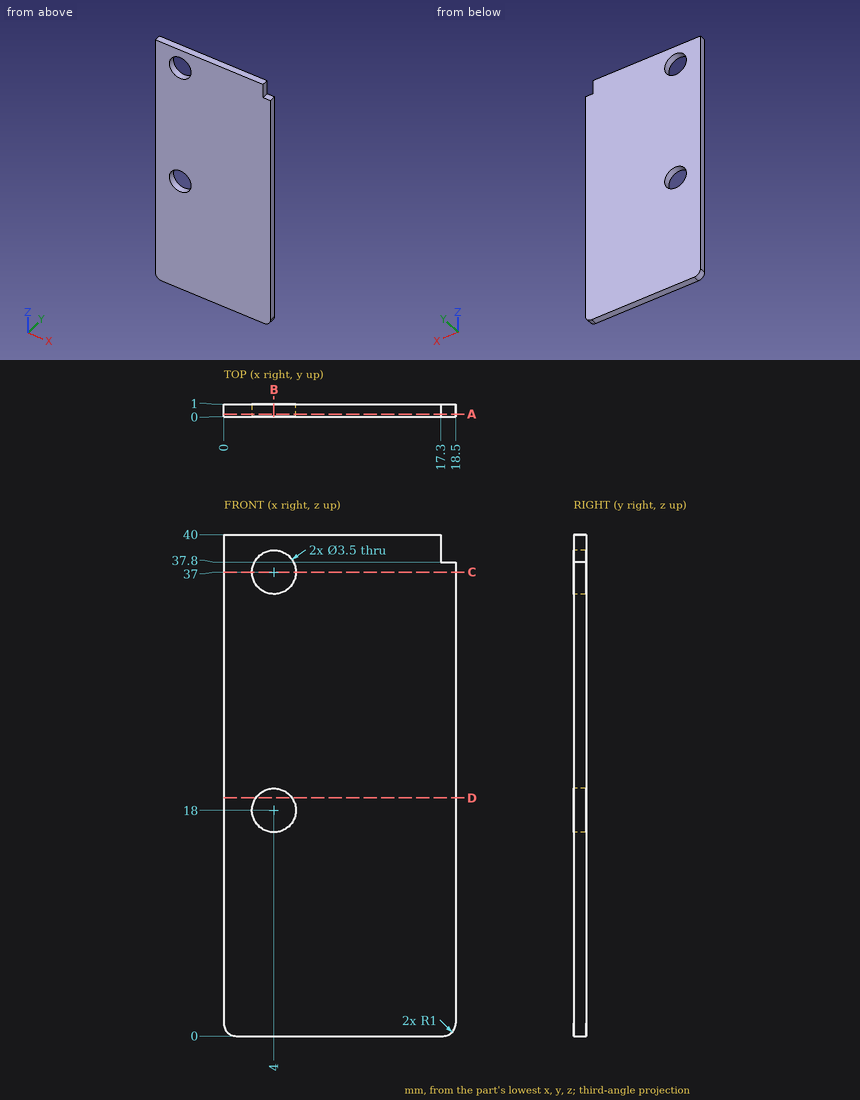
Print and shaded views of the part. All mm, measured from the part's lowest x, y and z. Give positions to 0.01 mm unless a question says otherwise; leave off trailing zeros. Write each loop counter-clockwise with the first axis right and the second up, starting at its lowest first coordinate (ties: lowest second). Pieces come first, ordered by that corner, then holes. Notation, with made-up numbers: (-13, 24) -> (30, 24) arc R11 ccw to (30, 34) -> close; hole circle Ø3 at (0.25, -2.5). An arc over 180 degrees is marked (long way). Write item = value, one per line.
(1) Slice it at B-B, the plane x = 4. Give the cut face in (y, z), then the cut area to 3 significant figures.
Determined:
outline = (0, 0) -> (1, 0) -> (1, 16.25) -> (0, 16.25) -> close; (0, 19.75) -> (1, 19.75) -> (1, 35.25) -> (0, 35.25) -> close; (0, 38.75) -> (1, 38.75) -> (1, 40) -> (0, 40) -> close
area = 33.0 mm2
(2) Slice it at D-D, the plane z = 19. Give the cut face in (x, y).
Determined:
outline = (0, 0) -> (2.56, 0) -> (2.56, 1) -> (0, 1) -> close; (5.44, 0) -> (18.5, 0) -> (18.5, 1) -> (5.44, 1) -> close
(3) Slice it at A-A, the plane y = 0.2. Give the cut face in (x, z), then the cut area to 3 significant figures.
Determined:
outline = (0, 1) arc R1 ccw to (1, 0) -> (17.5, 0) arc R1 ccw to (18.5, 1) -> (18.5, 37.8) -> (17.3, 37.8) -> (17.3, 40) -> (0, 40) -> close; hole circle Ø3.5 at (4, 18); hole circle Ø3.5 at (4, 37)
area = 718 mm2
(4) Flat gauge pin, fed straight in: P1, Ø2, axis at x = 4, z = 37, coming from the -Y side. Where does the tip first touch, or does it go through?
Determined:
P1 = through
(5) Probe line 1 along Z through (x, y) = (4, 0.7); line 2 along X through (y, z) = (0.3, 18); line 3 along Z through (x, y) = (5, 0.5). List the from-to ranges inside material, lowest first.
Determined:
line_1 = 0 to 16.25, 19.75 to 35.25, 38.75 to 40
line_2 = 0 to 2.25, 5.75 to 18.5
line_3 = 0 to 16.56, 19.44 to 35.56, 38.44 to 40
(6) Slice it at C-C, the plane z = 37. Give the cut face in (x, y), then the cut area to 3 significant figures.
Determined:
outline = (0, 0) -> (2.25, 0) -> (2.25, 1) -> (0, 1) -> close; (5.75, 0) -> (18.5, 0) -> (18.5, 1) -> (5.75, 1) -> close
area = 15.0 mm2
